```python
from build123d import *

# Parameters (mm, degrees)
F0_W     = 22
F0_H     = 70
F1_DEPTH = 2.5
F2_W     = 2
F2_H     = 70
F3_DEPTH = 3
F4_DEPTH = 9.5
F5_W     = 70
F5_H     = 2
F6_DEPTH = 3


with BuildPart() as f1:
    # F0 (on Top) → F1 (new body)
    with BuildSketch(Plane.XY):
        with Locations((-3.216149, -10.944109)):
            Rectangle(F0_W, F0_H)
    extrude(amount=F1_DEPTH)

    # F2 (on face) → F3 (join)
    with BuildSketch(Plane.XY.offset(2.5)):
        with Locations((-13.216149, -10.944109)):
            Rectangle(F2_W, F2_H)
    extrude(amount=F3_DEPTH)

    # F2 (on face) → F4 (join)
    with BuildSketch(Plane.XY.offset(2.5)):
        with Locations((6.783851, -10.944109)):
            Rectangle(F2_W, F2_H)
    extrude(amount=F4_DEPTH)

    # F5 (on face) → F6 (join)
    with BuildSketch(Plane(origin=(5.783851, 0, 0), x_dir=(0, -1, 0), z_dir=(-1, 0, 0))):
        with Locations((10.944109, 11)):
            Rectangle(F5_W, F5_H)
    extrude(amount=F6_DEPTH)


solid = f1.part
```
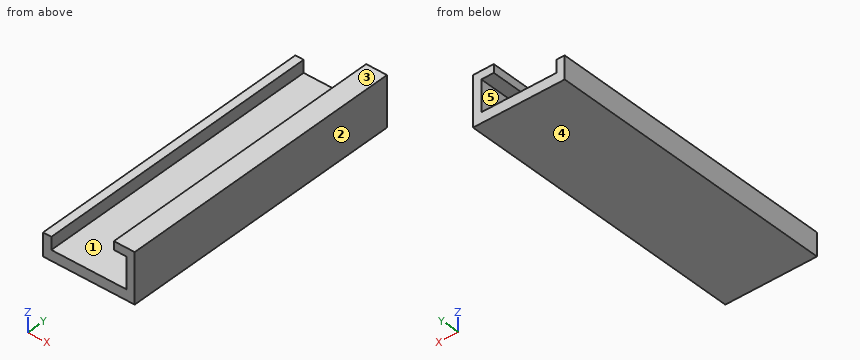
Read the model definition and answer for the solid it produces. Units are mm, in the model's axes. Face numbers are marked on the shaded views. A direction names the side the tool comes from. Coordinates: 2 decimals unless noted, no trailing zeros. Write each loop counter-clockwise with the first axis right and the second up, starting at its lowest first coordinate (ties: lowest second). Pieces come first, ordered by that corner, then holes. Notation, with made-up numbers: (36, 57) -> (75, 57) arc R16 cw to (75, 83) -> close; hole circle Ø2 at (-10, -32.5). An arc over 180 degrees is marked (long way). Answer as a JSON object with one key per item and string values.
Q1. Determine the mould class of the marked faces 1, 2 and 3 for opening direction X: pulls with the +X half, pulls with the -X half, needs draft (parallel to the pull), parting line crosses it, or undercut.
The answers:
{"face 1": "undercut", "face 2": "pulls with the +X half", "face 3": "needs draft"}
Q2. The part is cut by section C-C on y = -19. Give the vertices of the cut face in (x, z).
The answers:
{"outline": "(-14.22, 0) -> (7.78, 0) -> (7.78, 12) -> (2.78, 12) -> (2.78, 10) -> (5.78, 10) -> (5.78, 2.5) -> (-12.22, 2.5) -> (-12.22, 5.5) -> (-14.22, 5.5) -> close"}
Q3. Flat-ended cylindrical pins translate along their axes: pin 1 Ø9 at (x, y) = (-4, -20.5) entering from +Z; pin 2 Ø1.6 at (x, y) = (-13, -8) entering from +Z; pin 3 Ø5 at (x, z) = (-5, 5.5) entering from -Y; pin 4 Ø0.6 at (y, z) = (-17.5, 11.5) entering from -X. Find the tip coordinate at first contact, or state that the pin passes through.
The answers:
{"pin 1": "stops at z = 2.5", "pin 2": "stops at z = 5.5", "pin 3": "passes through", "pin 4": "stops at x = 2.78"}
Q4. Consider line 1 (X direction, y = -39, z = 2.75); line 2 (Z direction, x = 5, y = -41.5); line 3 (Z direction, x = -11.25, y = -37). Determine where each line is inside the solid, lowest interval first. Write a range as [from, to].
The answers:
{"line 1": "x = [-14.22, -12.22], [5.78, 7.78]", "line 2": "z = [0, 2.5], [10, 12]", "line 3": "z = [0, 2.5]"}
Q5. The part is cut by section B-B on z = 3.5. Give the vertices of the cut face in (x, y), then the cut area to 3 significant figures.
The answers:
{"outline": "(-14.22, -45.94) -> (-12.22, -45.94) -> (-12.22, 24.06) -> (-14.22, 24.06) -> close; (5.78, -45.94) -> (7.78, -45.94) -> (7.78, 24.06) -> (5.78, 24.06) -> close", "area": "280 mm2"}
Q6. The part is cut by section A-A on x = 5. Give the vertices of the cut face in (y, z), then the cut area to 3 significant figures.
The answers:
{"outline": "(-45.94, 0) -> (24.06, 0) -> (24.06, 2.5) -> (-45.94, 2.5) -> close; (-45.94, 10) -> (24.06, 10) -> (24.06, 12) -> (-45.94, 12) -> close", "area": "315 mm2"}
Q7. The part is cut by section D-D on x = -0.25. Give the vertices of the cut face in (y, z), then the cut area to 3 significant figures.
The answers:
{"outline": "(-45.94, 0) -> (24.06, 0) -> (24.06, 2.5) -> (-45.94, 2.5) -> close", "area": "175 mm2"}
Q8. A tool of negligible diameter and unlimited length cuts with its end or side. For the marked faces 4 and 5, from which of +Z, -Z, +X, -X, +Y, -Y can it reach the whole face along a straight path? Write none if from no direction.
The answers:
{"face 4": "-Z, +X, -X, +Y, -Y", "face 5": "+Y, -Y"}
